Geometry check sheet. Reference: the model listing, model coordinates, mm. A direction names the side the tool comes from. Round coordinates to 2 decimals unless told otherwise and drop trailing zeros. Write each loop counter-clockwise with the first axis right and the second up, starting at its lowest first coordinate (ties: lowest second). Pieces come first, ordered by that corner, then holes. Notation, with made-up numbers: M 27,63 L 35,63 A20 cw 35,68 Z; hole C 59.25,85 d2. An arc over 180 degrees is marked long. Put each result on its own line as item: value. Start each with the question number.
(1) Section check A-A on z = 0. Record the cut outline in (x, y), then the cut area to 3 significant figures.
(2) Material ranges on probe 1 along Y at (x, z) = (2.2, 0.55); probe 2 along Z at (x, y) = (0, 9), recorded low to high.
(3) Section check B-B on y = 11.25. Record the cut outline in (x, z), then the cut area to 3 significant figures.
(4) Tool access check on faces 1 (the cylindrical face through (0, 10, 2)), 2 (the flat face through (2.5, 22, 0)). Record the directions out of +Z, -Z, +X, -X, +Y, -Y that give a thin tool (end or side, any length) a straight path to the whole face; none if there is none.
(5) Gauge pin test, flat ends, axial feed: pin 1 (1 mm diameter, centred on x = 0.5, y = 7, fed in from +Z); pin 2 (1.5 mm diameter, centred on y = 18, z = 0.5, fed in from +X). Record the tip position at first contact, or that the pin passes through.
from build123d import *

# Parameters (mm, degrees)
SKETCH1_R           = 2
BOSS_EXTRUDE1_DEPTH = 20.7
BOSS_EXTRUDE2_DEPTH = 2
CHAMFER1_SIZE       = 0.5
FILLET1_R           = 0.2


with BuildPart() as part:
    # Sketch1 → Boss-Extrude1 (new body)
    with BuildSketch(Plane(origin=(0, 0, 0), x_dir=(1, 0, 0), z_dir=(0, 1, 0))):
        Circle(SKETCH1_R)
    extrude(amount=BOSS_EXTRUDE1_DEPTH)

    # Sketch2 → Boss-Extrude2 (add)
    with BuildSketch(Plane(origin=(0, 20.7, 0), x_dir=(1, 0, 0), z_dir=(0, 1, 0))):
        Polygon((0, 2.886751346), (-2.5, 1.443375673), (-2.5, -1.443375673), (0, -2.886751346), (2.5, -1.443375673), (2.5, 1.443375673), align=None)
    extrude(amount=BOSS_EXTRUDE2_DEPTH)

    # Chamfer1
    chamfer1_edges = [part.edges().sort_by_distance(p)[0] for p in [
        (-2, 0, 0),
    ]]
    chamfer(chamfer1_edges, length=CHAMFER1_SIZE)

    # Fillet1
    fillet1_edges = [part.edges().sort_by_distance(p)[0] for p in [
        (-2, 20.7, 0),
    ]]
    fillet(fillet1_edges, radius=FILLET1_R)


solid = part.part
Answers follow:
1. outline: M -2.5,20.7 L -2.2,20.7 A0.2 cw -2,20.5 L -2,0.5 L -1.5,0 L 1.5,0 L 2,0.5 L 2,20.5 A0.2 cw 2.2,20.7 L 2.5,20.7 L 2.5,22.7 L -2.5,22.7 Z
1. area: 92.6 mm^2
2. probe 1: y = 20.7 to 22.7
2. probe 2: z = -2 to 2
3. outline: C 0,0 d4
3. area: 12.6 mm^2
4. face 1: -Y
4. face 2: +Z, -Z, +X, +Y, -Y
5. pin 1: stops at z = 2
5. pin 2: stops at x = 2
